Work out the finished part from the listing and answer in its coordinate system (mm). A direction names the side the tool comes from. Coordinates: 2 decimals unless noted, no trailing zeros. Write each loop counter-clockwise with the first axis right and the second up, starting at its lowest first coordinate (ties: lowest second). Pieces come first, ordered by that corner, then holes. Notation, with made-up numbers: (34, 30) - (78, 30) arc R27 ccw to (78, 68) - close; hole circle Ø7 at (21.25, 26.5). An arc over 180 degrees is marked (long way). Use one line per item in the form item = value. Start each with the question number.
Item 1: Determine the mould class of faces 1 (the flat face through (2, 17.145, -9)), 2 (the cylindrical face through (-7.956, 8.452, -7.296)), 3 (the flat face through (1.744, 4.185, -6.51)) for opening direction Z: released by +Z, released by -Z, zero draft, split by the parting line, or undercut.
Item 2: A cutting plane is placed at C-C (z = 0). Write down the section's boundary in (x, y) (3 decimals).
Item 3: A cutting plane is placed at B-B (y = 6.25). Write down the section's boundary in (x, z) (3 decimals).
Item 4: Given pin 1 (3 mm diameter, centred on y = 6, z = 2, fed in from -X); pin 2 (1 mm diameter, centred on y = 12.5, z = 4, fed in from -X); pin 3 (6 mm diameter, centred on x = -7.5, y = 14.5, fed in from +Z); pin 4 (5.5 mm diameter, centred on x = -2, z = -2, fed in from +Y), each flat-ended and moving along its own axis, determine where each tip first touches the part or whether it passes through.
Item 5: Consider probe 1 along Z at (x, y) = (0, 14.5) (3 decimals); probe 2 along X at (y, z) = (11.1, 0) (3 decimals); probe 3 along X at (y, z) = (5.5, 0) (3 decimals). Determine where each line is inside the solid, lowest interval first.
Item 6: For faces 4 (the flat face through (5, 0, 5)), 5 (the cylindrical face through (-1.93, 15.27, 8.68)), determine the directions among +Z, -Z, +X, -X, +Y, -Y from which every point of the face is accessible in a straight line to the end or side of a thin tool.
Item 7: A cutting plane is placed at D-D (x = 3.75). Write down the section's boundary in (y, z) (3 decimals), then the cut area to 3 significant figures.
from build123d import *

# Parameters (mm, degrees)
SKETCH1_R           = 10.795
SKETCH1_R_2         = 6.096
BOSS_EXTRUDE1_DEPTH = 17.145
SKETCH2_R           = 8.89
CUT_EXTRUDE1_DEPTH  = 3.81
SKETCH3_R           = 7.366
SKETCH3_R_2         = 6.096
CUT_EXTRUDE2_DEPTH  = 5.08
CUT_EXTRUDE3_DEPTH  = 8.255


with BuildPart() as part:
    # Sketch1 → Boss-Extrude1 (new body)
    with BuildSketch(Plane(origin=(0, 0, 0), x_dir=(1, 0, 0), z_dir=(0, 1, 0))):
        Circle(SKETCH1_R)
        Circle(SKETCH1_R_2, mode=Mode.SUBTRACT)
    extrude(amount=BOSS_EXTRUDE1_DEPTH)

    # Sketch2 → Cut-Extrude1 (cut)
    with BuildSketch(Plane(origin=(0, 17.145, 0), x_dir=(1, 0, 0), z_dir=(0, 1, 0))):
        Circle(SKETCH2_R)
    extrude(amount=-CUT_EXTRUDE1_DEPTH, mode=Mode.SUBTRACT)

    # Sketch3 → Cut-Extrude2 (cut)
    with BuildSketch(Plane(origin=(0, 13.335, 0), x_dir=(1, 0, 0), z_dir=(0, 1, 0))):
        Circle(SKETCH3_R)
        Circle(SKETCH3_R_2, mode=Mode.SUBTRACT)
    extrude(amount=-CUT_EXTRUDE2_DEPTH, mode=Mode.SUBTRACT)

    # Sketch4 → Cut-Extrude3 (cut)
    with BuildSketch(Plane(origin=(0, 8.255, 0), x_dir=(1, 0, 0), z_dir=(0, 1, 0))):
        with BuildLine():
            Line((0, 0), (-1.906461086, 7.115009636))
            ThreePointArc((-1.906461086, 7.115009636), (0, 7.366), (1.906461086, 7.115009636))
            Line((1.906461086, 7.115009636), (0, 0))
        make_face()
    extrude(amount=-CUT_EXTRUDE3_DEPTH, mode=Mode.SUBTRACT)


solid = part.part
Answer:
q1.face_1 = zero draft
q1.face_2 = split by the parting line
q1.face_3 = undercut
q2.outline = (-10.795, 0) - (-6.096, 0) - (-6.096, 8.255) - (-7.366, 8.255) - (-7.366, 13.335) - (-8.89, 13.335) - (-8.89, 17.145) - (-10.795, 17.145) - close; (6.096, 0) - (10.795, 0) - (10.795, 17.145) - (8.89, 17.145) - (8.89, 13.335) - (7.366, 13.335) - (7.366, 8.255) - (6.096, 8.255) - close
q3.outline = circle Ø21.59 at (0, 0); hole (-1.906, -7.115) arc R7.366 ccw to (1.906, -7.115) - (1.578, -5.888) arc R6.096 ccw (long way) to (-1.578, -5.888) - close
q4.pin_1 = -10.78
q4.pin_2 = -10.21
q4.pin_3 = 9.81
q4.pin_4 = through
q5.probe_1 = -10.795 to -8.89, 8.89 to 10.795
q5.probe_2 = -10.795 to -7.366, 7.366 to 10.795
q5.probe_3 = -10.795 to -6.096, 6.096 to 10.795
q6.face_4 = +Z, -Z, +X, -X, -Y
q6.face_5 = +Y
q7.outline = (0, -10.123) - (17.145, -10.123) - (17.145, -8.06) - (13.335, -8.06) - (13.335, -6.34) - (8.255, -6.34) - (8.255, -4.806) - (0, -4.806) - close; (0, 4.806) - (8.255, 4.806) - (8.255, 6.34) - (13.335, 6.34) - (13.335, 8.06) - (17.145, 8.06) - (17.145, 10.123) - (0, 10.123) - close
q7.area = 142 mm²
